Part print with two shaded views. Sizes in mm from the minimum x, y, z corner. Round coordinates to 2 decimals unless told otherwise and drop trailing zeros. Order: outer loops, then holes, each group sorted by start corner. A loop starts at its lowest first (then second) coordinate and runs counter-clockwise, first axis right, second up. Notation, with made-up numbers: (78, 2.5) - (113, 2.5) arc R25 cw to (113, 40.5) - close; hole circle Ø10 at (9.25, 85.5). An arc over 180 degrees is marked (long way). Write item = value, one per line.
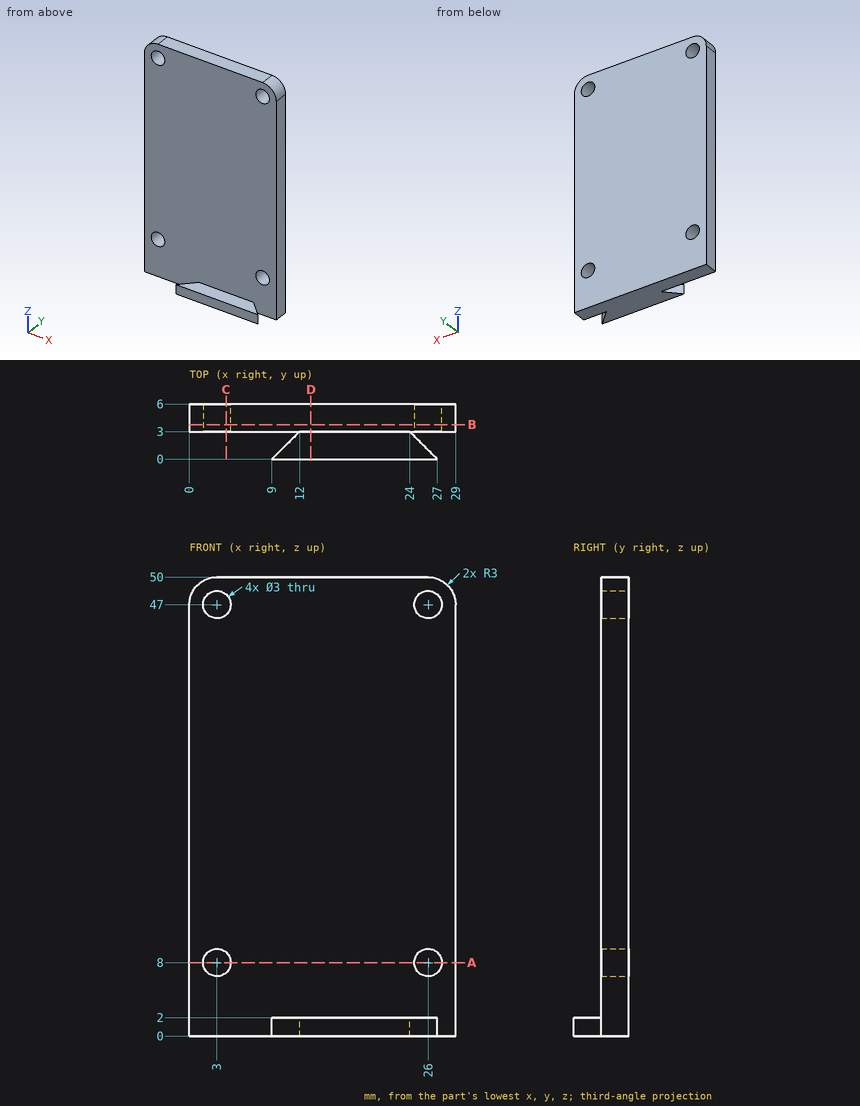
1) Cut at A-A (z = 8). Write the cut outline in (x, y).
Conclusion:
outline = (0, 3) - (1.5, 3) - (1.5, 6) - (0, 6) - close; (4.5, 3) - (24.5, 3) - (24.5, 6) - (4.5, 6) - close; (27.5, 3) - (29, 3) - (29, 6) - (27.5, 6) - close
2) Cut at C-C (x = 4). Write the cut outline in (y, z), and give its area (3 significant figures).
Conclusion:
outline = (3, 0) - (6, 0) - (6, 6.88) - (3, 6.88) - close; (3, 9.12) - (6, 9.12) - (6, 45.88) - (3, 45.88) - close; (3, 48.12) - (6, 48.12) - (6, 50) - (3, 50) - close
area = 137 mm^2
3) Wall check: line 1 along Z through (x, y) = (26, 4.05); line 2 along Y through (x, z) = (12.25, 31.5); line 3 along Z through (x, y) = (19.5, 1.05). Give the ranges that are in metal, low to high.
Conclusion:
line_1 = 0 to 6.5, 9.5 to 45.5, 48.5 to 50
line_2 = 3 to 6
line_3 = 0 to 2
4) Flat gauge pins, fed straight in: pin 1 Ø4 at (x, z) = (26, 8) entering from +Y; pin 2 Ø8 at (x, z) = (17, 43.5) entering from -Y; pin 3 Ø0.9 at (x, y) = (20.5, 1) entering from +Z. Where does each tip first touch, or does it go through?
Conclusion:
pin_1 = 6
pin_2 = 3
pin_3 = 2
5) Cut at D-D (x = 13.25). Write the cut outline in (y, z).
Conclusion:
outline = (0, 0) - (6, 0) - (6, 50) - (3, 50) - (3, 2) - (0, 2) - close
6) Cut at B-B (y = 3.75). Write the cut outline in (x, z).
Conclusion:
outline = (0, 0) - (29, 0) - (29, 47) arc R3 ccw to (26, 50) - (3, 50) arc R3 ccw to (0, 47) - close; hole circle Ø3 at (3, 8); hole circle Ø3 at (3, 47); hole circle Ø3 at (26, 8); hole circle Ø3 at (26, 47)
